Geometry check sheet. Reference: the model listing, model coordinates, mm. A direction names the side the tool comes from. Round coordinates to 2 decimals unless told otherwise and drop trailing zeros. Write each loop counter-clockwise with the first axis right and the second up, starting at its lowest first coordinate (ties: lowest second). Pieces come first, ordered by that corner, then holes. Notation, with made-up numbers: (24.25, 21) - (38.25, 21) arc R19 ccw to (38.25, 30) - close; hole circle Ø9 at (-31.75, 45). An arc over 180 degrees is marked (long way). Return JSON: item names as keys, results as strings. Group by question number.
from build123d import *

# Parameters (mm, degrees)
BOSS_EXTRUDE1_DEPTH     = 600
CUT_EXTRUDE1_DEPTH      = 743.024258364
CUT_EXTRUDE1_DEPTH_BACK = 743.024258364
CUT_EXTRUDE2_START      = -450
CUT_EXTRUDE2_DEPTH      = 450
FILLET1_R               = 200
SHELL2_START            = 53.190392924
SHELL2_OUTLINE_R        = 149
SHELL2_DEPTH            = 546.809607076
SHELL2_START_2          = 5.290187796
SHELL2_2_DEPTH          = 144.709812204


# Read off the part's stored shape, not the designer's step: Shell2
with BuildPart() as part:
    # Sketch1 → Boss-Extrude1 (new body)
    with BuildSketch(Plane(origin=(0, 0, 0), x_dir=(1, 0, 0), z_dir=(0, 1, 0))):
        with BuildLine():
            Line((8.485281374, -8.485281374), (150, -150))
            Line((150, -150), (260, -150))
            ThreePointArc((260, -150), (410, 0), (260, 150))
            Line((260, 150), (150, 150))
            Line((150, 150), (8.485281374, 8.485281374))
            ThreePointArc((8.485281374, 8.485281374), (12, 0), (8.485281374, -8.485281374))
        make_face()
    extrude(amount=BOSS_EXTRUDE1_DEPTH)

    # Sketch2 → Cut-Extrude1 (cut, two sides: drawn at the far end of the back side and taken through both)
    with BuildSketch(Plane.XY.offset(-CUT_EXTRUDE1_DEPTH_BACK)):
        Polygon((0, 0), (410, 236.713610368), (410, 0), align=None)
    extrude(amount=CUT_EXTRUDE1_DEPTH + CUT_EXTRUDE1_DEPTH_BACK, mode=Mode.SUBTRACT)

    # Sketch3 → Cut-Extrude2 (cut)
    with BuildSketch(Plane(origin=(0, 600, 0), x_dir=(1, 0, 0), z_dir=(0, 1, 0)).offset(CUT_EXTRUDE2_START)):
        with BuildLine():
            Line((0, 0), (150, 150))
            Line((150, 150), (260, 150))
            ThreePointArc((260, 150), (110, 0), (260, -150))
            Line((260, -150), (150, -150))
            Line((150, -150), (0, 0))
        make_face()
    extrude(amount=CUT_EXTRUDE2_DEPTH, mode=Mode.SUBTRACT)

    # Fillet1
    fillet1_edges = [part.edges().sort_by_distance(p)[0] for p in [
        (150, 118.301270189, 150),
        (150, 118.301270189, -150),
    ]]
    fillet(fillet1_edges, radius=FILLET1_R)

    # Shell2 outline → Shell2 (cut)
    with BuildSketch(Plane(origin=(0, 0, 0), x_dir=(1, 0, 0), z_dir=(0, 1, 0)).offset(SHELL2_START)):
        with Locations((260, 0)):
            Circle(SHELL2_OUTLINE_R)
    extrude(amount=SHELL2_DEPTH, mode=Mode.SUBTRACT)

    # Shell2 2 outline → Shell2 2 (cut)
    with BuildSketch(Plane(origin=(0, 0, 0), x_dir=(1, 0, 0), z_dir=(0, 1, 0)).offset(SHELL2_START_2)):
        with BuildLine():
            Line((9.162874044, -7.748660481), (92.128463018, -90.714249456))
            ThreePointArc((92.128463018, -90.714249456), (156.688709434, -133.85202697), (232.842712475, -149))
            Line((232.842712475, -149), (260, -149))
            ThreePointArc((260, -149), (111, 0), (260, 149))
            Line((260, 149), (232.842712475, 149))
            ThreePointArc((232.842712475, 149), (156.688709434, 133.85202697), (92.128463018, 90.714249456))
            Line((92.128463018, 90.714249456), (9.162874044, 7.748660481))
            ThreePointArc((9.162874044, 7.748660481), (12, 0), (9.162874044, -7.748660481))
        make_face()
    extrude(amount=SHELL2_2_DEPTH, mode=Mode.SUBTRACT)


solid = part.part
1. Depth check by flat-ended pin: pin 1 Ø1 at (y, z) = (183, 111.5) entering from +X; pin 2 Ø6 at (y, z) = (316.5, -92.5) entering from +X; pin 3 Ø1.5 at (y, z) = (322, -22) entering from -X. Enter the tip coordinate at first touch or a pass-through.
2. Mould release check, pull along Z, two halves, no side actions. Record for faces 4 (the face through (139.52, 112.87, -126.89)), 5 (the face through (139.99, 111.67, 126.01)), 6 (the face through (139.52, 112.87, 126.89)), 7 (the face through (111.276, 371.85, 19.527)): pulls with the +Z half, pulls with the -Z half, needs draft (parallel to the pull), parting line crosses it, or undercut.
3. Section check A-A (z = -124). Enter the section's corners in (x, y), and give its area (3 significant figures).
4. Material ranges on line 1 along Z through (x, y) = (260, 322); line 2 along X through (y, z) = (260, 0); line 3 along Z through (x, y) = (264, 520.5), recorded low to high.
5. Section check D-D (x = 149). Enter the section's corners in (y, z).
6. Tool access check on faces 1 (the face through (240, 146, 150)), 2 (the face through (141.93, 111.67, -127.02)), 3 (the face through (241, 146, -149)). Record the directions out of +Z, -Z, +X, -X, +Y, -Y that give a thin tool (end or side, any length) a straight path to the whole face; none if there is none.
7. Section check B-B (x = 282). Enter the section's corners in (y, z).
Result sheet:
{
 "1": {"pin 1": "stops at x = 161.73", "pin 2": "stops at x = 380.37", "pin 3": "stops at x = 111.51"},
 "2": {"face 4": "pulls with the -Z half", "face 5": "undercut", "face 6": "pulls with the +Z half", "face 7": "parting line crosses it"},
 "3": {"outline": "(134.23, 77.5) - (136.28, 78.68) - (136.28, 150) - (134.23, 150) - close; (175.6, 150) - (177.39, 150) - (177.39, 600) - (175.6, 600) - close; (342.61, 197.81) - (344.4, 198.84) - (344.4, 600) - (342.61, 600) - close", "area": "1,670 mm²"},
 "4": {"line 1": "z = -150 to -149, 149 to 150", "line 2": "x = 110 to 111, 409 to 410", "line 3": "z = -149.95 to -148.95, 148.95 to 149.95"},
 "5": {"outline": "(86.03, -131.58) - (150, -131.58) - (150, -130.48) - (86.03, -130.48) - close; (86.03, 130.48) - (150, 130.48) - (150, 131.58) - (86.03, 131.58) - close; (150, -100.89) - (600, -100.89) - (600, -99.4) - (150, -99.4) - close; (150, 99.4) - (600, 99.4) - (600, 100.89) - (150, 100.89) - close"},
 "6": {"face 1": "+Z, +X, -X, +Y, -Y", "face 2": "+X, +Y, -Y", "face 3": "+X, -Y"},
 "7": {"outline": "(162.81, -148.38) - (600, -148.38) - (600, -147.37) - (162.81, -147.37) - close; (162.81, 147.37) - (600, 147.37) - (600, 148.38) - (162.81, 148.38) - close"}
}
